```python
from build123d import *

# Parameters (mm, degrees)
F0_W      = 80
F0_H      = 30
F1_DEPTH  = 6
F3_DEPTH  = 6.001
F4_W      = 20
F4_H      = 16
F5_DEPTH  = 20
F6_W      = 11.27
F6_H      = 14.08
F7_DEPTH  = 18
F8_R      = 2.97
F9_DEPTH  = 62.001
F10_W     = 10
F10_H     = 9
F11_DEPTH = 9
F12_R     = 1.55
F13_DEPTH = 19.501
F14_W     = 20
F14_H     = 5
F15_DEPTH = 19
F16_W     = 20
F16_H     = 4
F17_DEPTH = 25
F18_R     = 1.55
F19_DEPTH = 4


with BuildPart() as f1:
    # F0 (on Top) → F1 (new body)
    with BuildSketch(Plane.XY):
        Rectangle(F0_W, F0_H)
    extrude(amount=F1_DEPTH)

    # F2 (on face) → F3 (cut, through all)
    with BuildSketch(Plane.XY.offset(6)):
        with BuildLine():
            Line((35.55, -7.5), (35.55, 7.5))
            ThreePointArc((35.55, 7.5), (33, 10.05), (30.45, 7.5))
            Line((30.45, 7.5), (30.45, -7.5))
            ThreePointArc((30.45, -7.5), (33, -10.05), (35.55, -7.5))
        make_face()
        with BuildLine():
            Line((-4.45, -7.5), (-4.45, 7.5))
            ThreePointArc((-4.45, 7.5), (-7, 10.05), (-9.55, 7.5))
            Line((-9.55, 7.5), (-9.55, -7.5))
            ThreePointArc((-9.55, -7.5), (-7, -10.05), (-4.45, -7.5))
        make_face()
    extrude(amount=-F3_DEPTH, mode=Mode.SUBTRACT)

    # F4 (on face) → F5 (join)
    with BuildSketch(Plane.XY.offset(6)):
        with Locations((-30, 0)):
            Rectangle(F4_W, F4_H)
    extrude(amount=F5_DEPTH)

    # F6 (on face) → F7 (cut)
    with BuildSketch(Plane(origin=(-40, 0, 0), x_dir=(0, -1, 0), z_dir=(-1, 0, 0))):
        with Locations((0, 15.96)):
            Rectangle(F6_W, F6_H)
    extrude(amount=-F7_DEPTH, mode=Mode.SUBTRACT)

    # F8 (on face) → F9 (cut, through all)
    with BuildSketch(Plane(origin=(-22, 0, 0), x_dir=(0, -1, 0), z_dir=(-1, 0, 0))):
        with Locations((0, 15.96)):
            Circle(F8_R)
    extrude(amount=-F9_DEPTH, mode=Mode.SUBTRACT)

    # F10 (on face) → F11 (join)
    with BuildSketch(Plane.XY.offset(26)):
        with Locations((-29, 0)):
            Rectangle(F10_W, F10_H)
    extrude(amount=F11_DEPTH)

    # F12 (on face) → F13 (cut, through all)
    with BuildSketch(Plane.XZ.offset(4.5)):
        with Locations((-29, 30.5)):
            Circle(F12_R)
    extrude(amount=-F13_DEPTH, mode=Mode.SUBTRACT)

    # F14 (on face) → F15 (cut)
    with BuildSketch(Plane.XY.offset(35)):
        with Locations((-30, 0)):
            Rectangle(F14_W, F14_H)
    extrude(amount=-F15_DEPTH, mode=Mode.SUBTRACT)

    # F16 (on Top) → F17 (join)
    with BuildSketch(Plane.XY):
        with Locations((-30, -12)):
            Rectangle(F16_W, F16_H)
    extrude(amount=F17_DEPTH)

    # F18 (on face) → F19 (cut)
    with BuildSketch(Plane.XZ.offset(14)):
        with Locations((-36, 20.29)):
            Circle(F18_R)
        with Locations((-36, 11.99)):
            Circle(F18_R)
        with Locations((-29, 20.29)):
            Circle(F18_R)
        with Locations((-29, 11.99)):
            Circle(F18_R)
    extrude(amount=-F19_DEPTH, mode=Mode.SUBTRACT)


solid = f1.part
```
Build history of the part. All positions in model axes, mm. A direction names the side the tool comes from. Round coordinates to 2 decimals unless told otherwise and drop trailing zeros. Write each loop counter-clockwise with the first axis right and the second up, starting at its lowest first coordinate (ties: lowest second). Pieces come first, ordered by that corner, then holes. Notation, with made-up numbers: (56.25, 15) - (113.25, 15) arc R12 ccw to (113.25, 24) - close; hole circle Ø5 at (8.5, 0). An arc over 180 degrees is marked (long way). Write each question's results on one line, items separated by ' | '. Start each with the question number.
Item 1: Wall check: L1, parallel to Z at x = -29, y = -4; L2, parallel to Z at x = -36, y = -12.8; L3, parallel to X at y = 5.5, z = 2.5. Give the ranges that are in metal, low to high. Write a range as [from, to].
Item 2: Saw through at A-A (z = 11.99). Write the cut outline in (x, y) (3 decimals), and give its area (3 significant figures).
Item 3: Saw through at B-B (y = -6.75). Write the cut outline in (x, z).
Item 4: Saw through at C-C (x = -36). Write the cut outline in (y, z) (3 decimals).
Item 5: Saw through at D-D (z = 15.96). Write the cut outline in (x, y) (3 decimals), and give its area (3 significant figures).
Item 6: Mould opens along Z. For faces 1 (the face through (-27.568, -12.028, 11.396)), 2 (the face through (-29, 4, 35)), 3 (the face through (-4.45, 0, 3)), 4 (the face through (-28.17, 3.49, 31.81)) say: pulls with the +Z half, pulls with the -Z half, needs draft (parallel to the pull), parting line crosses it, or undercut.
Item 7: Which spindle directions (+Z, -Z, +X, -X, +Y, -Y) get a long thin tool onto all of the face, cutting with end or side? Do faces 5 (the face through (-35.17, -12.03, 21.6)), 6 (the face through (-31, 4, 23)), 7 (the face through (-34, 3, 30)). Say none if no direction does.
Item 8: Drop flat-ended pins along their axis: P1, Ø17.5, axis at y = 2.5, z = 17, coming from the +X side; P2, Ø5, axis at x = -29, z = 27.5, coming from the +Y side; P3, Ø9.5, axis at x = -28.5, z = 18.5, coming from the -Y side. Give the stop position or say it passes through.
Results are:
1) L1: z = [0, 8.92], [23, 28.95], [32.05, 35] | L2: z = [0, 10.44], [13.54, 18.74], [21.84, 25] | L3: x = [-40, -9.55], [-4.45, 30.45], [35.55, 40]
2) outline: (-40, -14) - (-37.55, -14) - (-37.55, -10) - (-40, -10) - close; (-40, -8) - (-20, -8) - (-20, 8) - (-40, 8) - (-40, 5.635) - (-22, 5.635) - (-22, -5.635) - (-40, -5.635) - close; (-34.45, -14) - (-30.55, -14) - (-30.55, -10) - (-34.45, -10) - close; (-27.45, -14) - (-20, -14) - (-20, -10) - (-27.45, -10) - close | area: 172 mm²
3) outline: (-40, 0) - (-9.55, 0) - (-9.55, 6) - (-20, 6) - (-20, 26) - (-40, 26) - close; (-4.45, 0) - (30.45, 0) - (30.45, 6) - (-4.45, 6) - close; (35.55, 0) - (40, 0) - (40, 6) - (35.55, 6) - close
4) outline: (-15, 0) - (15, 0) - (15, 6) - (8, 6) - (8, 26) - (2.5, 26) - (2.5, 23) - (5.635, 23) - (5.635, 8.92) - (-5.635, 8.92) - (-5.635, 23) - (-2.5, 23) - (-2.5, 26) - (-8, 26) - (-8, 6) - (-10, 6) - (-10, 10.44) - (-14, 10.44) - (-14, 6) - (-15, 6) - close; (-14, 13.54) - (-10, 13.54) - (-10, 18.74) - (-14, 18.74) - close; (-14, 21.84) - (-10, 21.84) - (-10, 25) - (-14, 25) - close
5) outline: (-40, -14) - (-20, -14) - (-20, -10) - (-40, -10) - close; (-40, -8) - (-20, -8) - (-20, -2.97) - (-22, -2.97) - (-22, -5.635) - (-40, -5.635) - close; (-40, 5.635) - (-22, 5.635) - (-22, 2.97) - (-20, 2.97) - (-20, 8) - (-40, 8) - close | area: 185 mm²
6) face 1: undercut | face 2: pulls with the +Z half | face 3: needs draft | face 4: undercut
7) face 5: -Y | face 6: -X | face 7: +Z, -X, +Y, -Y
8) P1: stops at x = -20 | P2: stops at y = 8 | P3: stops at y = -14
